```python
from build123d import *

# Parameters (mm, degrees)
F0_R     = 11
F2_DEPTH = 3.175
F1_R     = 11
F3_DEPTH = 12.7


with BuildPart() as f2:
    # F0 (on Front) → F2 (new body, symmetric)
    with BuildSketch(Plane.XZ):
        with BuildLine():
            ThreePointArc((-7.2482056801, 14.3587687297), (-6.5765724866, 16.6617776341), (-6.35, 19.05))
            ThreePointArc((-6.35, 19.05), (-29.5587734092, 26.1813169495), (-14.3587687297, 7.2482056801))
            add(Edge.make_bspline(
                [(-14.3587687297, 7.2482056801), (-15.3619108037, 10.3222858149), (-16.9256545604, 14.0228222828), (-19.05, 19.05)],
                knots=[28.0456445655, 28.0456445655, 28.0456445655, 28.0456445655, 38.1, 38.1, 38.1, 38.1], degree=3))
            add(Edge.make_bspline(
                [(-19.05, 19.05), (-14.0228222828, 16.9256545604), (-10.3222858149, 15.3619108037), (-7.2482056801, 14.3587687297)],
                knots=[0, 0, 0, 0, 10.0543554345, 10.0543554345, 10.0543554345, 10.0543554345], degree=3))
        make_face()
        with BuildLine():
            add(Edge.make_bspline(
                [(-14.3587687297, 7.2482056801), (-15.3619108037, 10.3222858149), (-16.9256545604, 14.0228222828), (-19.05, 19.05)],
                knots=[28.0456445655, 28.0456445655, 28.0456445655, 28.0456445655, 38.1, 38.1, 38.1, 38.1], degree=3))
            ThreePointArc((-14.3587687297, 7.2482056801), (-10.0697438789, 10.0697438789), (-7.2482056801, 14.3587687297))
            add(Edge.make_bspline(
                [(-19.05, 19.05), (-14.0228222828, 16.9256545604), (-10.3222858149, 15.3619108037), (-7.2482056801, 14.3587687297)],
                knots=[0, 0, 0, 0, 10.0543554345, 10.0543554345, 10.0543554345, 10.0543554345], degree=3))
        make_face()
        with BuildLine():
            ThreePointArc((-7.2482056801, 14.3587687297), (-10.0697438789, 10.0697438789), (-14.3587687297, 7.2482056801))
            add(Edge.make_bspline(
                [(-14.3587687297, -7.2482056801), (-12.5637437568, -1.7474388854), (-12.5637437568, 1.7474388854), (-14.3587687297, 7.2482056801)],
                knots=[10.0543554345, 10.0543554345, 10.0543554345, 10.0543554345, 28.0456445655, 28.0456445655, 28.0456445655, 28.0456445655], degree=3))
            ThreePointArc((-14.3587687297, -7.2482056801), (-10.0697438789, -10.0697438789), (-7.2482056801, -14.3587687297))
            add(Edge.make_bspline(
                [(-7.2482056801, -14.3587687297), (-1.7474388854, -12.5637437568), (1.7474388854, -12.5637437568), (7.2482056801, -14.3587687297)],
                knots=[10.0543554345, 10.0543554345, 10.0543554345, 10.0543554345, 28.0456445655, 28.0456445655, 28.0456445655, 28.0456445655], degree=3))
            ThreePointArc((7.2482056801, -14.3587687297), (10.0697438789, -10.0697438789), (14.3587687297, -7.2482056801))
            add(Edge.make_bspline(
                [(14.3587687297, 7.2482056801), (12.5637437568, 1.7474388854), (12.5637437568, -1.7474388854), (14.3587687297, -7.2482056801)],
                knots=[10.0543554345, 10.0543554345, 10.0543554345, 10.0543554345, 28.0456445655, 28.0456445655, 28.0456445655, 28.0456445655], degree=3))
            ThreePointArc((14.3587687297, 7.2482056801), (10.0697438789, 10.0697438789), (7.2482056801, 14.3587687297))
            add(Edge.make_bspline(
                [(-7.2482056801, 14.3587687297), (-1.7474388854, 12.5637437568), (1.7474388854, 12.5637437568), (7.2482056801, 14.3587687297)],
                knots=[10.0543554345, 10.0543554345, 10.0543554345, 10.0543554345, 28.0456445655, 28.0456445655, 28.0456445655, 28.0456445655], degree=3))
        make_face()
        Circle(F0_R, mode=Mode.SUBTRACT)
        with BuildLine():
            add(Edge.make_bspline(
                [(-19.05, -19.05), (-16.9256545604, -14.0228222828), (-15.3619108037, -10.3222858149), (-14.3587687297, -7.2482056801)],
                knots=[0, 0, 0, 0, 10.0543554345, 10.0543554345, 10.0543554345, 10.0543554345], degree=3))
            ThreePointArc((-14.3587687297, -7.2482056801), (-29.5587734092, -26.1813169495), (-6.35, -19.05))
            ThreePointArc((-6.35, -19.05), (-6.5765724866, -16.6617776341), (-7.2482056801, -14.3587687297))
            add(Edge.make_bspline(
                [(-19.05, -19.05), (-14.0228222828, -16.9256545604), (-10.3222858149, -15.3619108037), (-7.2482056801, -14.3587687297)],
                knots=[0, 0, 0, 0, 10.0543554345, 10.0543554345, 10.0543554345, 10.0543554345], degree=3))
        make_face()
        with BuildLine():
            ThreePointArc((-7.2482056801, -14.3587687297), (-10.0697438789, -10.0697438789), (-14.3587687297, -7.2482056801))
            add(Edge.make_bspline(
                [(-19.05, -19.05), (-16.9256545604, -14.0228222828), (-15.3619108037, -10.3222858149), (-14.3587687297, -7.2482056801)],
                knots=[0, 0, 0, 0, 10.0543554345, 10.0543554345, 10.0543554345, 10.0543554345], degree=3))
            add(Edge.make_bspline(
                [(-19.05, -19.05), (-14.0228222828, -16.9256545604), (-10.3222858149, -15.3619108037), (-7.2482056801, -14.3587687297)],
                knots=[0, 0, 0, 0, 10.0543554345, 10.0543554345, 10.0543554345, 10.0543554345], degree=3))
        make_face()
        with BuildLine():
            add(Edge.make_bspline(
                [(7.2482056801, 14.3587687297), (10.3222858149, 15.3619108037), (14.0228222828, 16.9256545604), (19.05, 19.05)],
                knots=[28.0456445655, 28.0456445655, 28.0456445655, 28.0456445655, 38.1, 38.1, 38.1, 38.1], degree=3))
            ThreePointArc((7.2482056801, 14.3587687297), (10.0697438789, 10.0697438789), (14.3587687297, 7.2482056801))
            add(Edge.make_bspline(
                [(19.05, 19.05), (16.9256545604, 14.0228222828), (15.3619108037, 10.3222858149), (14.3587687297, 7.2482056801)],
                knots=[0, 0, 0, 0, 10.0543554345, 10.0543554345, 10.0543554345, 10.0543554345], degree=3))
        make_face()
        with BuildLine():
            ThreePointArc((31.75, 19.05), (16.6617776341, 31.5234275134), (7.2482056801, 14.3587687297))
            add(Edge.make_bspline(
                [(7.2482056801, 14.3587687297), (10.3222858149, 15.3619108037), (14.0228222828, 16.9256545604), (19.05, 19.05)],
                knots=[28.0456445655, 28.0456445655, 28.0456445655, 28.0456445655, 38.1, 38.1, 38.1, 38.1], degree=3))
            add(Edge.make_bspline(
                [(19.05, 19.05), (16.9256545604, 14.0228222828), (15.3619108037, 10.3222858149), (14.3587687297, 7.2482056801)],
                knots=[0, 0, 0, 0, 10.0543554345, 10.0543554345, 10.0543554345, 10.0543554345], degree=3))
            ThreePointArc((14.3587687297, 7.2482056801), (26.1813169495, 8.5412265908), (31.75, 19.05))
        make_face()
        with BuildLine():
            add(Edge.make_bspline(
                [(7.2482056801, -14.3587687297), (10.3222858149, -15.3619108037), (14.0228222828, -16.9256545604), (19.05, -19.05)],
                knots=[28.0456445655, 28.0456445655, 28.0456445655, 28.0456445655, 38.1, 38.1, 38.1, 38.1], degree=3))
            ThreePointArc((7.2482056801, -14.3587687297), (16.6617776341, -31.5234275134), (31.75, -19.05))
            ThreePointArc((31.75, -19.05), (26.1813169495, -8.5412265908), (14.3587687297, -7.2482056801))
            add(Edge.make_bspline(
                [(14.3587687297, -7.2482056801), (15.3619108037, -10.3222858149), (16.9256545604, -14.0228222828), (19.05, -19.05)],
                knots=[28.0456445655, 28.0456445655, 28.0456445655, 28.0456445655, 38.1, 38.1, 38.1, 38.1], degree=3))
        make_face()
        with BuildLine():
            ThreePointArc((14.3587687297, -7.2482056801), (10.0697438789, -10.0697438789), (7.2482056801, -14.3587687297))
            add(Edge.make_bspline(
                [(7.2482056801, -14.3587687297), (10.3222858149, -15.3619108037), (14.0228222828, -16.9256545604), (19.05, -19.05)],
                knots=[28.0456445655, 28.0456445655, 28.0456445655, 28.0456445655, 38.1, 38.1, 38.1, 38.1], degree=3))
            add(Edge.make_bspline(
                [(14.3587687297, -7.2482056801), (15.3619108037, -10.3222858149), (16.9256545604, -14.0228222828), (19.05, -19.05)],
                knots=[28.0456445655, 28.0456445655, 28.0456445655, 28.0456445655, 38.1, 38.1, 38.1, 38.1], degree=3))
        make_face()
    extrude(amount=F2_DEPTH, both=True)

    # F1 (on Front) → F3 (cut, symmetric)
    with BuildSketch(Plane.XZ):
        with Locations((-19.0500058234, 19.0502889454)):
            Circle(F1_R)
        with Locations((19.0496798605, 19.0498717129)):
            Circle(F1_R)
        with Locations((-19.0505106002, -19.0498437732)):
            Circle(F1_R)
        with Locations((19.0585404634, -19.0461371094)):
            Circle(F1_R)
    extrude(amount=F3_DEPTH, both=True, mode=Mode.SUBTRACT)


solid = f2.part
```
Can you work these out from the model? Positions are in its coordinate system, mm. Coordinates: 2 decimals unless noted, no trailing zeros. Loops run counter-clockwise (first coordinate to the right, second up) from the corner with the lowest first, then second, coordinate; pieces in that order, holes last.
1) Thinking about a two-plate mould opening in Z: for faces 1 (the flat face through (12, 3.175, 0)), 2 (the cylindrical face through (16.674, -0.044, -29.785)), which applies, pulls with the +Z half, pulls with the -Z half, needs draft (parallel to the pull), parting line crosses it, or undercut?
2) For pin 1 (2 mm diameter, centred on x = -17.5, y = -1, fed in from -Z); pin 2 (10 mm diameter, centred on x = -10.5, z = 17.5, fed in from -Y) (3 decimals); pin 3 (3 mm diameter, centred on x = -4.5, y = 0, fed in from -Z), each with a flat end and sliding along its axis, tell me the tip position at first contact or that it passes through.
3) Imagine slicing it at C-C on y = -2. State how many separate pieces and enclosed holes the cut face has, plus the area to 3 significant figures.
4) Imagine slicing it at A-A on x = 22.5. List the corners of the cut face in (y, z) for me (3 decimals), plus the area to 3 significant figures.
5) I need wall thicknesses on probe 1 along Z at (x, y) = (0, -2.3); probe 2 along X at (y, z) = (0.25, -27.5); probe 3 along Z at (x, y) = (26, 1.5). Which ranges of each line are inside material? Lowest first, please.
6) Imagine slicing it at B-B on z = -23. List the corners of the cut face in (x, y) for me (3 decimals), plus the area to 3 significant figures.
Completed:
1. face 1: needs draft
1. face 2: undercut
2. pin 1: stops at z = -31.74
2. pin 2: stops at y = -3.175
2. pin 3: stops at z = -13.97
3. separate pieces: 1
3. enclosed holes: 5
3. area: 771 mm2
4. outline: (-3.175, -31.272) - (3.175, -31.272) - (3.175, -29.494) - (-3.175, -29.494) - close; (-3.175, -8.598) - (3.175, -8.598) - (3.175, -6.828) - (-3.175, -6.828) - close; (-3.175, 6.828) - (3.175, 6.828) - (3.175, 8.605) - (-3.175, 8.605) - close; (-3.175, 29.495) - (3.175, 29.495) - (3.175, 31.272) - (-3.175, 31.272) - close
4. area: 45.1 mm2
5. probe 1: z = -13.01 to -11, 11 to 13.01
5. probe 2: x = -28.53 to -26.09, -12.01 to -9.57, 9.57 to 12.02, 26.1 to 28.53
5. probe 3: z = -29.68 to -27.58, -10.51 to -8.42, 8.42 to 10.52, 27.58 to 29.68
6. outline: (-31.12, -3.175) - (-29.317, -3.175) - (-29.317, 3.175) - (-31.12, 3.175) - close; (-8.784, -3.175) - (-6.98, -3.175) - (-6.98, 3.175) - (-8.784, 3.175) - close; (6.98, -3.175) - (8.794, -3.175) - (8.794, 3.175) - (6.98, 3.175) - close; (29.323, -3.175) - (31.12, -3.175) - (31.12, 3.175) - (29.323, 3.175) - close
6. area: 45.8 mm2
